Model file for the job. Use its own axes, mm. Face numbers are marked on the shaded views. A direction names the side the tool comes from. Round coordinates to 2 decimals unless told otherwise and drop trailing zeros. Write each loop counter-clockwise with the first axis right and the second up, starting at its lowest first coordinate (ties: lowest second). Pieces come first, ordered by that corner, then holes. Notation, with made-up numbers: (3, -22) - (37, -22) arc R23 cw to (37, -7) - close; hole circle Ø9 at (52, 11). An arc over 180 degrees is marked (long way). One line per item, written item: value.
from build123d import *

# Parameters (mm, degrees)
SKETCH1_W           = 27.94
SKETCH1_H           = 27.94
BOSS_EXTRUDE1_DEPTH = 127
CUT_EXTRUDE1_REACH  = 130.528
SKETCH2_W           = 22.86
SKETCH2_H           = 22.86
SKETCH3_W           = 50.8
SKETCH3_H           = 177.8
BOSS_EXTRUDE2_DEPTH = 10.16
CUT_EXTRUDE2_REACH  = 221.622
SKETCH4_R           = 6.35
SKETCH5_W           = 177.8
SKETCH5_H           = 10.16
BOSS_EXTRUDE3_DEPTH = 203.2
SKETCH7_R           = 7.5
CUT_EXTRUDE4_DEPTH  = 5.08


with BuildPart() as part:
    # Sketch1 → Boss-Extrude1 (new body)
    with BuildSketch(Plane(origin=(0, 0, 0), x_dir=(1, 0, 0), z_dir=(0, 1, 0))):
        Rectangle(SKETCH1_W, SKETCH1_H)
    extrude(amount=BOSS_EXTRUDE1_DEPTH)

    # Sketch2 → Cut-Extrude1 (cut, up to next)
    with BuildSketch(Plane(origin=(0, 127, 0), x_dir=(1, 0, 0), z_dir=(0, 1, 0)), mode=Mode.PRIVATE) as cut_extrude1_sk1:
        Rectangle(SKETCH2_W, SKETCH2_H)
    cut_extrude1_tool1 = extrude(cut_extrude1_sk1.sketch, amount=-CUT_EXTRUDE1_REACH, mode=Mode.PRIVATE) & part.part
    add(cut_extrude1_tool1.solids().sort_by_distance((0, 127, 0))[0], mode=Mode.SUBTRACT)

    # Sketch3 → Boss-Extrude2 (add)
    with BuildSketch(Plane(origin=(0, 127, 0), x_dir=(1, 0, 0), z_dir=(0, 1, 0))):
        with Locations((-11.43, -74.93)):
            Rectangle(SKETCH3_W, SKETCH3_H)
    extrude(amount=BOSS_EXTRUDE2_DEPTH)

    # Sketch4 → Cut-Extrude2 (cut, up to next)
    with BuildSketch(Plane(origin=(13.97, 0, 0), x_dir=(0, 0, -1), z_dir=(1, 0, 0)), mode=Mode.PRIVATE) as cut_extrude2_sk1:
        with Locations((0, 25.4)):
            Circle(SKETCH4_R)
    cut_extrude2_tool1 = extrude(cut_extrude2_sk1.sketch, amount=-CUT_EXTRUDE2_REACH, mode=Mode.PRIVATE) & part.part
    # Sketch4 → Cut-Extrude2 (cut, up to next)
    with BuildSketch(Plane(origin=(13.97, 0, 0), x_dir=(0, 0, -1), z_dir=(1, 0, 0)), mode=Mode.PRIVATE) as cut_extrude2_sk2:
        with Locations((0, 43.18)):
            Circle(SKETCH4_R)
    cut_extrude2_tool2 = extrude(cut_extrude2_sk2.sketch, amount=-CUT_EXTRUDE2_REACH, mode=Mode.PRIVATE) & part.part
    # Sketch4 → Cut-Extrude2 (cut, up to next)
    with BuildSketch(Plane(origin=(13.97, 0, 0), x_dir=(0, 0, -1), z_dir=(1, 0, 0)), mode=Mode.PRIVATE) as cut_extrude2_sk3:
        with Locations((0, 60.96)):
            Circle(SKETCH4_R)
    cut_extrude2_tool3 = extrude(cut_extrude2_sk3.sketch, amount=-CUT_EXTRUDE2_REACH, mode=Mode.PRIVATE) & part.part
    # Sketch4 → Cut-Extrude2 (cut, up to next)
    with BuildSketch(Plane(origin=(13.97, 0, 0), x_dir=(0, 0, -1), z_dir=(1, 0, 0)), mode=Mode.PRIVATE) as cut_extrude2_sk4:
        with Locations((0, 78.74)):
            Circle(SKETCH4_R)
    cut_extrude2_tool4 = extrude(cut_extrude2_sk4.sketch, amount=-CUT_EXTRUDE2_REACH, mode=Mode.PRIVATE) & part.part
    # Sketch4 → Cut-Extrude2 (cut, up to next)
    with BuildSketch(Plane(origin=(13.97, 0, 0), x_dir=(0, 0, -1), z_dir=(1, 0, 0)), mode=Mode.PRIVATE) as cut_extrude2_sk5:
        with Locations((0, 96.52)):
            Circle(SKETCH4_R)
    cut_extrude2_tool5 = extrude(cut_extrude2_sk5.sketch, amount=-CUT_EXTRUDE2_REACH, mode=Mode.PRIVATE) & part.part
    add(cut_extrude2_tool1.solids().sort_by_distance((13.97, 25.4, 0))[0], mode=Mode.SUBTRACT)
    add(cut_extrude2_tool2.solids().sort_by_distance((13.97, 43.18, 0))[0], mode=Mode.SUBTRACT)
    add(cut_extrude2_tool3.solids().sort_by_distance((13.97, 60.96, 0))[0], mode=Mode.SUBTRACT)
    add(cut_extrude2_tool4.solids().sort_by_distance((13.97, 78.74, 0))[0], mode=Mode.SUBTRACT)
    add(cut_extrude2_tool5.solids().sort_by_distance((13.97, 96.52, 0))[0], mode=Mode.SUBTRACT)

    # Sketch5 → Boss-Extrude3 (add)
    with BuildSketch(Plane(origin=(13.97, 0, 0), x_dir=(0, 0, -1), z_dir=(1, 0, 0))):
        with Locations((-74.93, 132.08)):
            Rectangle(SKETCH5_W, SKETCH5_H)
    extrude(amount=BOSS_EXTRUDE3_DEPTH)

    # Sketch7 → Cut-Extrude4 (cut)
    with BuildSketch(Plane.XZ.offset(-127)):
        with Locations(Location((90.17, 43.501665218, 0), (0, 0, 270))):
            Circle(SKETCH7_R)
    extrude(amount=-CUT_EXTRUDE4_DEPTH, mode=Mode.SUBTRACT)


solid = part.part
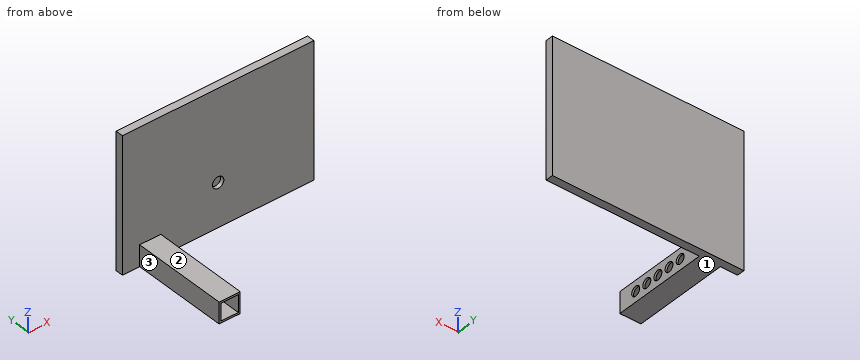
1. Band-saw the part on B-B on z = 0. State how many separate pieces and enclosed holes the cut face has, plus the area to 3 significant figures.
Report:
separate pieces: 6
enclosed holes: 0
area: 3,060 mm²
2. Band-saw the part on D-D on x = 90.17. Write the cut outline in (y, z).
Report:
outline: (127, -13.97) - (137.16, -13.97) - (137.16, 163.83) - (127, 163.83) - (127, 51) - (132.08, 51) - (132.08, 36) - (127, 36) - close
3. Drop flat-ended pins along their axis: pin 1 (11.5 mm diameter, centred on y = 60.96, z = 0, fed in from +X); pin 2 (2 mm diameter, centred on x = 136.5, z = 52.5, fed in from -Y); pin 3 (14.5 mm diameter, centred on y = 43.18, z = 0, fed in from -X); pin 4 (25 mm diameter, centred on x = 4, z = 2.5, fed in from -Y). Give the stop position or say it passes through.
Report:
pin 1: x = -11.43
pin 2: y = 127
pin 3: x = -13.97
pin 4: y = 0
4. Band-saw the part on C-C on y = 60.96. Write the cut outline in (x, z), plus the area to 3 significant figures.
Report:
outline: (-13.97, -13.97) - (13.97, -13.97) - (13.97, -6.35) - (11.43, -6.35) - (11.43, -11.43) - (-11.43, -11.43) - (-11.43, 11.43) - (11.43, 11.43) - (11.43, 6.35) - (13.97, 6.35) - (13.97, 13.97) - (-13.97, 13.97) - close
area: 226 mm²
5. Tool access for the marked faces 1, 2 and 3: list every direction of +Z, -Z, +X, -X, +Y, -Y with a clear straight run to the whole face (end or side of a thin tool).
Report:
face 1: -Z, +X, -X, +Y, -Y
face 2: +Z, +X, -X, -Y
face 3: +Z, -Z, -X, -Y
6. Wall check: probe 1 along Y at (x, z) = (12.6, 0); probe 2 along Z at (x, y) = (90, 130); probe 3 along X at (y, z) = (126.5, 7.5). Give the ranges that are in metal, low to high. Write a range as [from, to].
Report:
probe 1: [0, 19.05], [31.75, 36.83], [49.53, 54.61], [67.31, 72.39], [85.09, 90.17], [102.87, 137.16]
probe 2: [-13.97, 36], [51, 163.83]
probe 3: [-13.97, -11.43], [11.43, 13.97]
7. Band-saw the part on A-A on y = 107.5. Write the cut outline in (x, z), plus the area to 3 significant figures.
Report:
outline: (-13.97, -13.97) - (13.97, -13.97) - (13.97, 13.97) - (-13.97, 13.97) - close; hole (-11.43, -11.43) - (11.43, -11.43) - (11.43, 11.43) - (-11.43, 11.43) - close
area: 258 mm²
